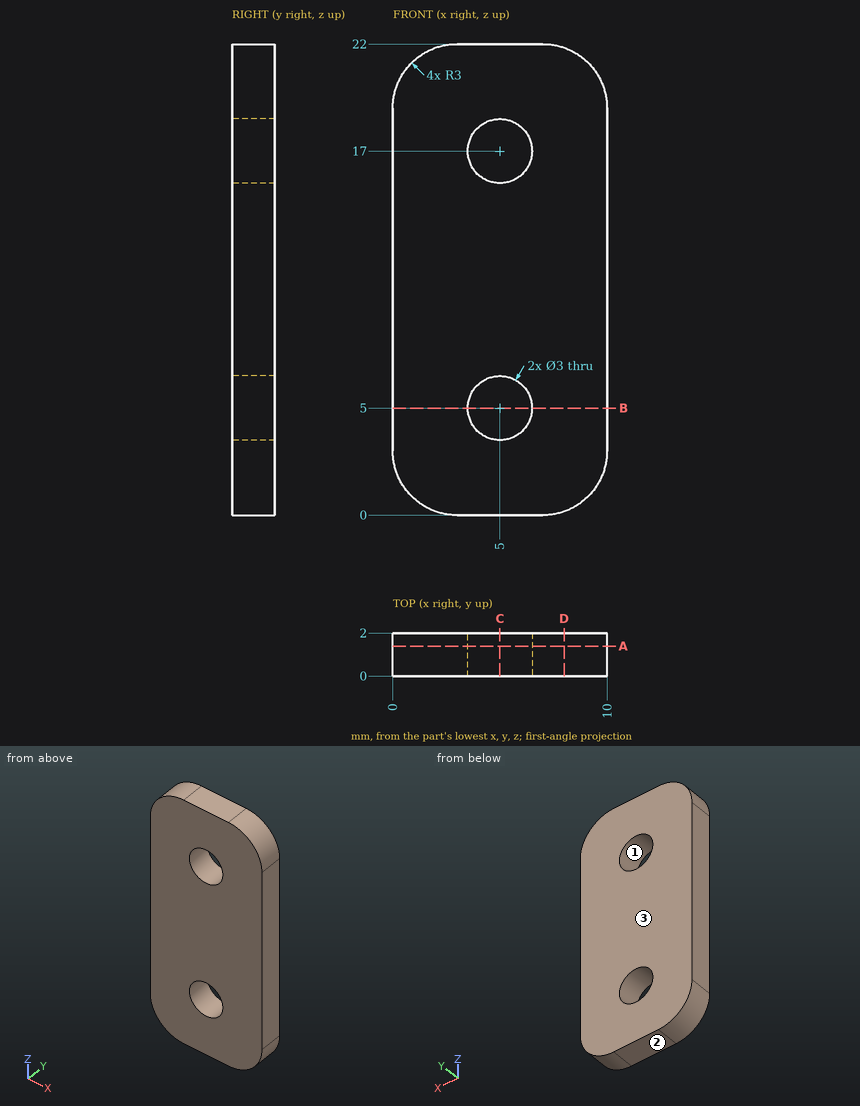
Study the drawing (mm; zero at the part's minimum x, y, z) and answer. Give positions to 0.01 mm unless a question says otherwise; leave off trailing zeros. Write each loop counter-clockwise with the first axis right and the second up, starting at its lowest first coordinate (ties: lowest second). Pieces come first, ordered by that corner, then holes. Notation, with made-up numbers: (62.5, 31.25) - (83.5, 31.25) arc R16 cw to (83.5, 39.25) - close; hole circle Ø8 at (-19, -19). An arc over 180 degrees is marked (long way). Use CSV: the item, a comma, the result in double quotes. Start each with the question number.
(1) Consider line 1 along Z through (x, y) = (5, 1.2); line 2 along Z through (x, y) = (6, 1.8); line 3 along X through (y, z) = (0.7, 16). Determine where each line is inside the solid, lowest interval first.
(2) Find section D-D (x = 8). Give the vertices of the cut face in (y, z).
(3) Determine the mould class of the marked faces 1, 2 and 3 for opening direction Z: +Z half, -Z half, draft (parallel to the pull), parting line (faces both ways), or undercut.
(4) Find section B-B (z = 5). Give the vertices of the cut face in (x, y).
(5) Find section C-C (x = 5). Give the vertices of the cut face in (y, z), plus the area to 3 significant figures.
(6) Find section A-A (y = 1.4). Give the vertices of the cut face in (x, z).
Findings below:
1,line 1,"0 to 3.5, 6.5 to 15.5, 18.5 to 22"
1,line 2,"0 to 3.88, 6.12 to 15.88, 18.12 to 22"
1,line 3,"0 to 3.88, 6.12 to 10"
2,outline,"(0, 0.17) - (2, 0.17) - (2, 21.83) - (0, 21.83) - close"
3,face 1,"undercut"
3,face 2,"-Z half"
3,face 3,"draft"
4,outline,"(0, 0) - (3.5, 0) - (3.5, 2) - (0, 2) - close; (6.5, 0) - (10, 0) - (10, 2) - (6.5, 2) - close"
5,outline,"(0, 0) - (2, 0) - (2, 3.5) - (0, 3.5) - close; (0, 6.5) - (2, 6.5) - (2, 15.5) - (0, 15.5) - close; (0, 18.5) - (2, 18.5) - (2, 22) - (0, 22) - close"
5,area,"32.0 mm2"
6,outline,"(0, 3) arc R3 ccw to (3, 0) - (7, 0) arc R3 ccw to (10, 3) - (10, 19) arc R3 ccw to (7, 22) - (3, 22) arc R3 ccw to (0, 19) - close; hole circle Ø3 at (5, 5); hole circle Ø3 at (5, 17)"
